Part model, mm, in its own coordinate system. A direction names the side the tool comes from. Give positions to 0.01 mm unless a question says otherwise; leave off trailing zeros. Order: outer loops, then holes, each group sorted by start corner. A loop starts at its lowest first (then second) coordinate and runs counter-clockwise, first axis right, second up. Notation, with made-up numbers: M -10.5,74.5 L -3.5,74.5 A12 ccw -3.5,97.5 Z; hole C -0.75,-7 d3. An arc over 180 degrees is marked long. Return JSON: item names as keys, results as strings.
from build123d import *

# Parameters (mm, degrees)
ESBO_O1_R                = 50.8
ESBO_O1_R_2              = 47.8
EXTRUS_O_FINA1_DEPTH     = 50
ESBO_O2_W                = 150
ESBO_O2_H                = 135
RESSALTO_EXTRUS_O1_DEPTH = 3
FILETE1_R                = 10
FILETE2_R                = 15
ESBO_O3_R                = 47.8
CORTE_EXTRUS_O1_DEPTH    = 113.611056296


with BuildPart() as part:
    # Esboço1 → Extrusão-Fina1 (new body)
    with BuildSketch(Plane(origin=(0, 0, 0), x_dir=(1, 0, 0), z_dir=(0, 1, 0))):
        Circle(ESBO_O1_R)
        Circle(ESBO_O1_R_2, mode=Mode.SUBTRACT)
    extrude(amount=EXTRUS_O_FINA1_DEPTH)

    # Esboço2 → Ressalto-extrusão1 (add)
    with BuildSketch(Plane.XZ):
        Rectangle(ESBO_O2_W, ESBO_O2_H)
    extrude(amount=RESSALTO_EXTRUS_O1_DEPTH)

    # Filete1
    filete1_edges = [part.edges().sort_by_distance(p)[0] for p in [
        (-50.8, 0, 0),
    ]]
    fillet(filete1_edges, radius=FILETE1_R)

    # Filete2
    filete2_edges = [part.edges().sort_by_distance(p)[0] for p in [
        (-75, -1.5, -67.5),
        (75, -1.5, -67.5),
        (75, -1.5, 67.5),
        (-75, -1.5, 67.5),
    ]]
    fillet(filete2_edges, radius=FILETE2_R)

    # Esboço3 → Corte-extrusão1 (cut, through all)
    with BuildSketch(Plane(origin=(0, 0, 0), x_dir=(1, 0, 0), z_dir=(0, 1, 0))):
        Circle(ESBO_O3_R)
    extrude(amount=-CORTE_EXTRUS_O1_DEPTH, mode=Mode.SUBTRACT)


solid = part.part
Q1. Two-plate mould, pull along Y, no slides. Class faces 3 (the flat face through (-34, 50, 34)), 4 (the flat face through (16, -3, 46)), 5 (the cylindrical face through (70.49, -1.52, -63.22)): +Y half, -Y half, draft (parallel to the pull), parting line (faces both ways), or undercut.
Established:
{"face 3": "+Y half", "face 4": "-Y half", "face 5": "draft"}
Q2. Band-saw the part on B-B (x = 0). Give the cut face in (y, z), then the cut area to 3 significant figures.
Established:
{"outline": "M -3,-67.5 L 0,-67.5 L 0,-60.8 A10 cw 10,-50.8 L 50,-50.8 L 50,-47.8 L -3,-47.8 Z; M -3,47.8 L 50,47.8 L 50,50.8 L 10,50.8 A10 cw 0,60.8 L 0,67.5 L -3,67.5 Z", "area": "461 mm²"}
Q3. 3-axis set-ups, long thin cutter, end or side, ignore diameter. For faces 1 (the flat face through (-1, 0, 61)), 2 (the cylindrical face through (70.49, -1.52, 63.22)): which of +Z, -Z, +X, -X, +Y, -Y reach the whole face in a straight line?
Established:
{"face 1": "+Y", "face 2": "+Z, +X, +Y, -Y"}
Q4. Band-saw the part on A-A (z = 0). Give the cut face in (x, y), then the cut area to 3 significant figures.
Established:
{"outline": "M -75,-3 L -47.8,-3 L -47.8,50 L -50.8,50 L -50.8,10 A10 cw -60.8,0 L -75,0 Z; M 47.8,-3 L 75,-3 L 75,0 L 60.8,0 A10 cw 50.8,10 L 50.8,50 L 47.8,50 Z", "area": "506 mm²"}
Q5. Pin check, flat tips, straight feed: pin 1 (4 mm diameter, centred on x = 21.5, y = 3, fed in from +Z); pin 2 (8 mm diameter, centred on x = 10.5, y = 26.5, fed in from -Z); pin 3 (2 mm diameter, centred on x = 10.5, y = 22, fed in from -Z). Stop position of each tip, or through.
Established:
{"pin 1": "stops at z = 52.26", "pin 2": "stops at z = -50.38", "pin 3": "stops at z = -49.9"}
Q6. Band-saw the part on C-C (y = 22.5). Give the cut face in (x, z), then the cut area to 3 significant figures.
Established:
{"outline": "C 0,0 d101.6; hole C 0,0 d95.6", "area": "929 mm²"}
Q7. Probe line 1 along X through (y, z) = (16, 0); line 2 along Z through (x, y) = (0, -1.85); line 3 along X through (y, z) = (-0.75, 0). List the from-to ranges inside material, lowest first.
Established:
{"line 1": "x = -50.8 to -47.8, 47.8 to 50.8", "line 2": "z = -67.5 to -47.8, 47.8 to 67.5", "line 3": "x = -75 to -47.8, 47.8 to 75"}
